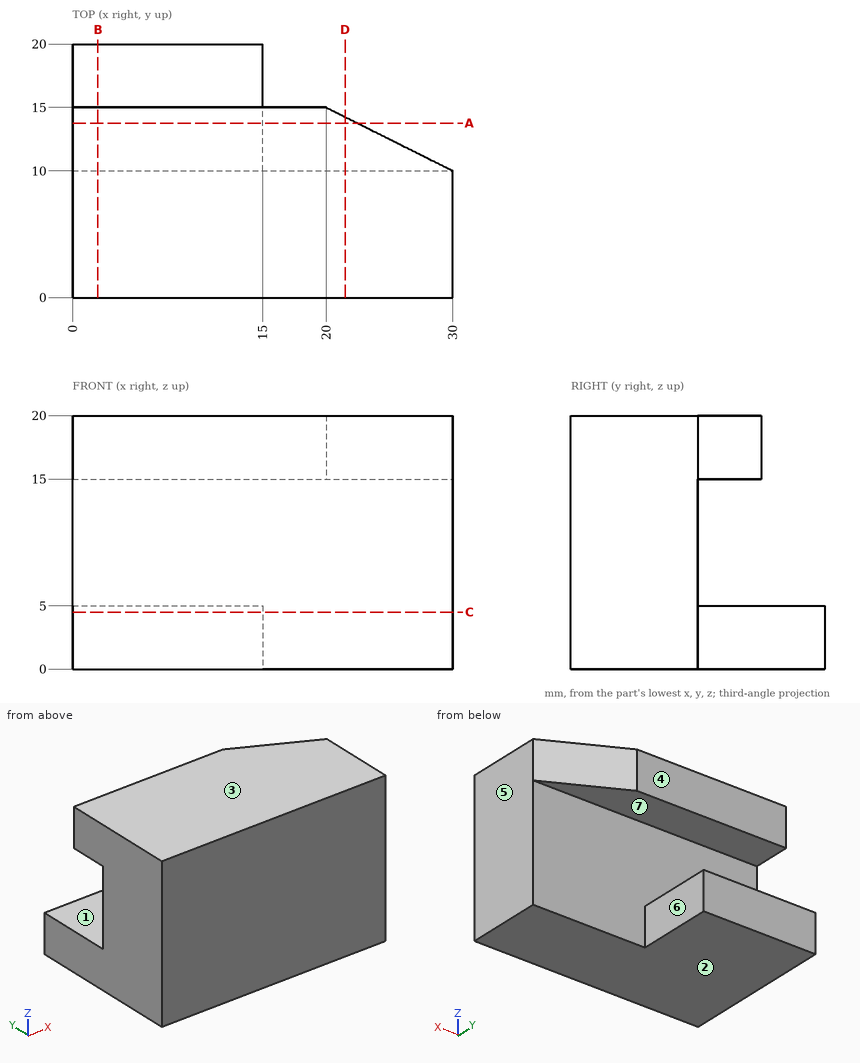
Geometry check sheet. Reference: drawing and pictorial views, mm from the part's lowest x, y, z. A direction names the side the tool comes from. Give positions to 0.01 mm unless a question says otherwise; leave off trailing zeros. Write each loop counter-clockwise with the first axis right and the second up, starting at its lowest first coordinate (ties: lowest second). Pieces come first, ordered by that corner, then holes. Notation, with made-up numbers: M 10.5,-18.5 L 15.5,-18.5 A20 ccw 15.5,1.5 Z; hole C 56.5,-40 d8. An arc over 180 degrees is marked long. Use CSV: the item, a comma, the result in double quotes.
1) Cross-section at C-C (z = 4.5). Enter the section's corners in (x, y).
Final values:
outline,"M 0,0 L 30,0 L 30,10 L 15,10 L 15,20 L 0,20 Z"
2) Cross-section at B-B (x = 2). Enter the section's corners in (y, z), plus the area to 3 significant figures.
Final values:
outline,"M 0,0 L 20,0 L 20,5 L 10,5 L 10,15 L 15,15 L 15,20 L 0,20 Z"
area,"275 mm²"
3) Go/stop test with flat-tipped pins: pin 1 Ø1 at (y, z) = (12, 6.5) entering from -X; pin 2 Ø5.5 at (y, z) = (14, 2) entering from +X; pin 3 Ø7.5 at (x, z) = (20, 6.5) entering from +Y; pin 4 Ø1.5 at (x, z) = (14, 17) entering from +Y. Record where each tip stops, or that it passes through.
Final values:
pin 1,"through"
pin 2,"x = 15"
pin 3,"y = 10"
pin 4,"y = 15"
4) Access from +Z, -Z, +X, -X, +Y, -Y to the whole of each face (thin tool, end or side, straight path). Record for the marked faces 5, 6 and 7.
Final values:
face 5,"+Z, -Z, +X, +Y, -Y"
face 6,"-Z, +X, +Y"
face 7,"+X, -X, +Y"
5) Cross-section at A-A (y = 13.75). Enter the section's corners in (x, z).
Final values:
outline,"M 0,0 L 15,0 L 15,5 L 0,5 Z; M 0,15 L 22.5,15 L 22.5,20 L 0,20 Z"
6) Cross-section at D-D (x = 21.5). Enter the section's corners in (y, z).
Final values:
outline,"M 0,0 L 10,0 L 10,15 L 14.25,15 L 14.25,20 L 0,20 Z"
7) Material ranges on line 1 along Z through (x, y) = (5, 11.5); line 2 along Y through (x, z) = (16, 9.25); line 3 along Y through (x, z) = (18.5, 17.25), recorded low to high.
Final values:
line 1,"0 to 5, 15 to 20"
line 2,"0 to 10"
line 3,"0 to 15"
8) Release check for a two-part mould opening along Z. For the marked faces 1, 2, 3 and 4 record: released by +Z, released by -Z, zero draft, split by the parting line, or undercut.
Final values:
face 1,"undercut"
face 2,"released by -Z"
face 3,"released by +Z"
face 4,"zero draft"
